Design review of the part shown in the three views and the two pictorial views. Dimensions are in mm from the part's minimum x, y and z. Coordinates: 2 decimals unless noted, no trailing zeros. Write each loop counter-clockwise with the first axis right and the second up, starting at its lowest first coordinate (ties: lowest second). Pieces come first, ordered by that corner, then holes. Notation, with made-up numbers: (-10, 60.25) -> (7, 60.25) arc R18 ccw to (7, 67.25) -> close; hole circle Ø10 at (25.25, -34). An arc over 180 degrees is marked (long way). Answer in a Markdown table with one row per item. Add a question column.
Item 1: To check wall thickness, follow line 1 (X direction, y = 2.05, z = 7.5); line 2 (Z direction, x = 24, y = 2.3); line 3 (Z direction, x = 49, y = 2.1). State the ranges of each line that lie inside material, in increasing order.
Item 2: Take a section at C-C, the plane x = 51.25. Write out the cut boundary in (y, z).
Item 3: Clearance check with flat-ended pins moving along their axes: P1, Ø1.5, axis at x = 52.5, y = 1, coming from the -Z side; P2, Ø1.5, axis at x = 44, y = 2, coming from the +Z side; P3, Ø0.9, axis at y = 1, z = 34.5, coming from the -X side. State where each tip first meets the part, or that it passes through.
Item 4: Take a section at D-D, the plane z = 7.5. Write out the cut boundary in (x, y).
Item 5: Take a section at A-A, the plane z = 53.75. Write out the cut boundary in (x, y).
Item 6: Take a section at B-B, the plane x = 5. Write out the cut boundary in (y, z), and give its area (3 significant figures).
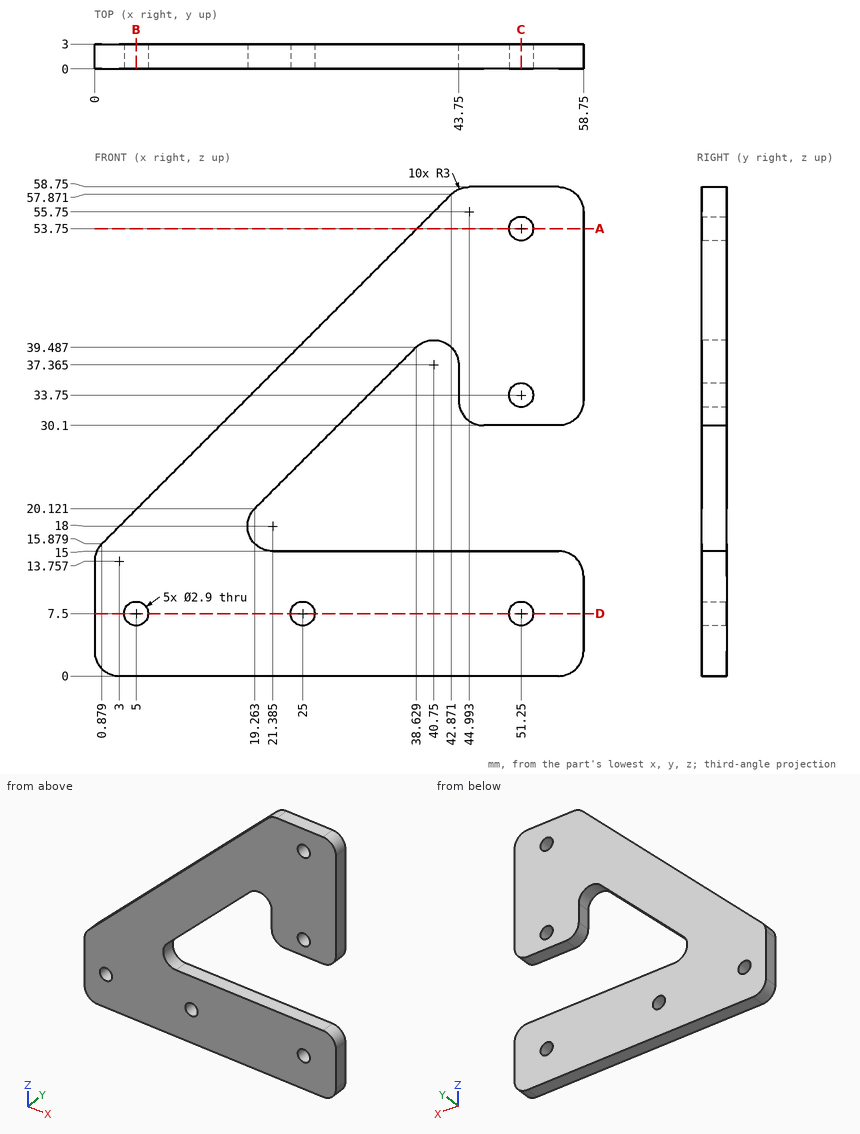
Answers:
| question | item | result |
|---|---|---|
| 1 | line 1 | x = 0 to 3.55, 6.45 to 23.55, 26.45 to 49.8, 52.7 to 58.75 |
| 1 | line 2 | z = 0 to 6.45, 8.55 to 15, 24.86 to 39 |
| 1 | line 3 | z = 0 to 15, 30.1 to 58.75 |
| 2 | outline | (0, 0) -> (3, 0) -> (3, 6.05) -> (0, 6.05) -> close; (0, 8.95) -> (3, 8.95) -> (3, 15) -> (0, 15) -> close; (0, 30.1) -> (3, 30.1) -> (3, 32.3) -> (0, 32.3) -> close; (0, 35.2) -> (3, 35.2) -> (3, 52.3) -> (0, 52.3) -> close; (0, 55.2) -> (3, 55.2) -> (3, 58.75) -> (0, 58.75) -> close |
| 3 | P1 | stops at z = 0 |
| 3 | P2 | stops at z = 58.74 |
| 3 | P3 | stops at x = 19.05 |
| 4 | outline | (0, 0) -> (3.55, 0) -> (3.55, 3) -> (0, 3) -> close; (6.45, 0) -> (23.55, 0) -> (23.55, 3) -> (6.45, 3) -> close; (26.45, 0) -> (49.8, 0) -> (49.8, 3) -> (26.45, 3) -> close; (52.7, 0) -> (58.75, 0) -> (58.75, 3) -> (52.7, 3) -> close |
| 5 | outline | (38.75, 0) -> (49.8, 0) -> (49.8, 3) -> (38.75, 3) -> close; (52.7, 0) -> (58.75, 0) -> (58.75, 3) -> (52.7, 3) -> close |
| 6 | outline | (0, 0) -> (3, 0) -> (3, 6.05) -> (0, 6.05) -> close; (0, 8.95) -> (3, 8.95) -> (3, 20) -> (0, 20) -> close |
| 6 | area | 51.3 mm^2 |
